Here's the drawing with two shaded views (mm, measured from the low corner). I have some questions. Give positions to 0.01 mm unless a question says otherwise; leave off trailing zeros. Loops run counter-clockwise (first coordinate to the right, second up) from the corner with the lowest first, then second, coordinate; pieces in that order, holes last. Notation, with made-up numbers: (82, 45) - (86, 45) arc R26 ccw to (86, 61) - close; hole circle Ø8 at (11, 35.5). An arc over 180 degrees is marked (long way). Write each question's results on one line, items separated by ' | '. Start each with the question number.
1) I want a section at A-A, the plane z = 54.94. Write out the boundary of the cut face in (x, y), and give its area (4 significant figures).
2) I want a section at B-B, the plane y = 5. Write out the boundary of the cut face in (x, z).
3) I'm going to push a flat-ended pin straight in: pin 1 (4 mm diameter, centred on y = 5, z = 5, fed in from -X). Where does the tip first touch, or does it pass through?
4) If I drill on probe 1 along Y at (x, z) = (2.7, 5); probe 2 along Z at (x, y) = (1.9, 155); probe 3 along Y at (x, z) = (2.75, 54.94), over which ranges is the centre line in solid material (lowest first)? Write a range as [from, to].
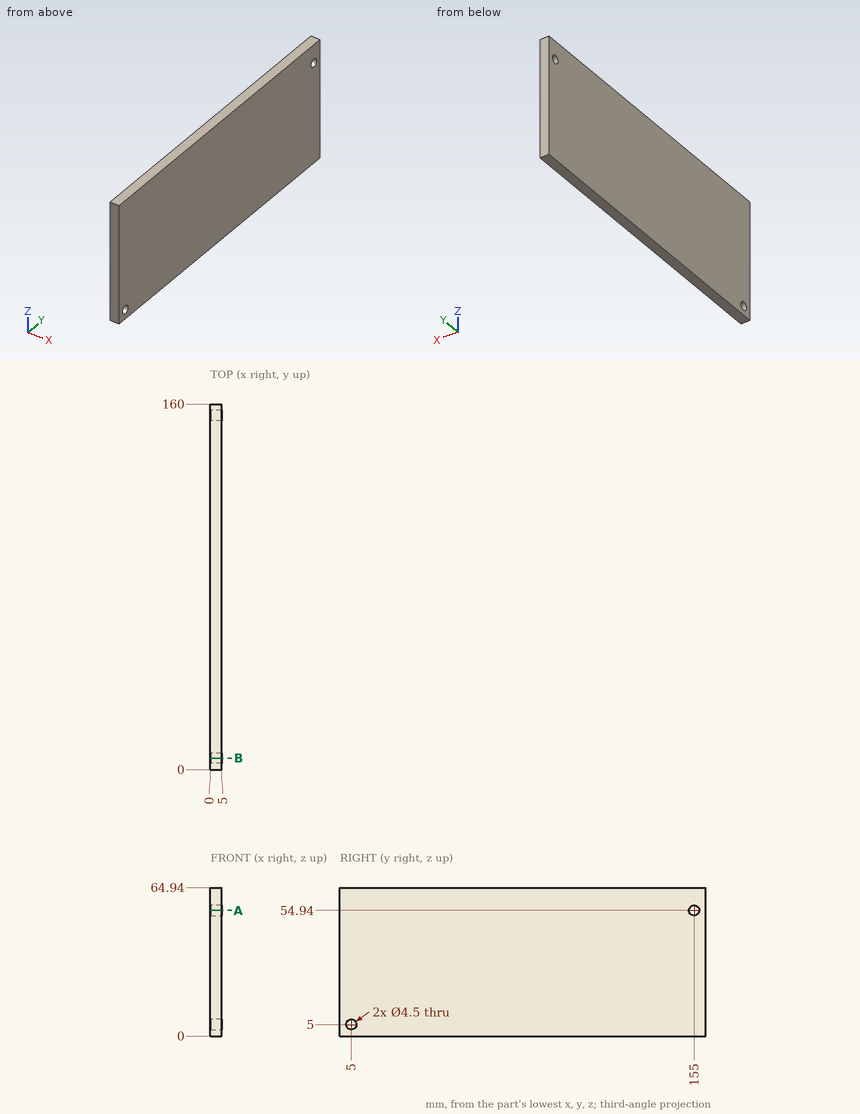
Answers:
1) outline: (0, 0) - (5, 0) - (5, 152.75) - (0, 152.75) - close; (0, 157.25) - (5, 157.25) - (5, 160) - (0, 160) - close | area: 777.5 mm2
2) outline: (0, 0) - (5, 0) - (5, 2.75) - (0, 2.75) - close; (0, 7.25) - (5, 7.25) - (5, 64.94) - (0, 64.94) - close
3) pin 1: passes through
4) probe 1: y = [0, 2.75], [7.25, 160] | probe 2: z = [0, 52.69], [57.19, 64.94] | probe 3: y = [0, 152.75], [157.25, 160]
